```python
from build123d import *

# Parameters (mm, degrees)
BOSS_EXTRUDE1_DEPTH  = 46.3
SKETCH3_R            = 11.25
CUT_EXTRUDE2_DEPTH   = 2
SKETCH3_5_R          = 1.5
SKETCH3_5_R_2        = 3
CUT_EXTRUDE3_DEPTH   = 5
SKETCH4_R            = 2
CUT_EXTRUDE4_DEPTH   = 5
SKETCH5_W            = 5
SKETCH5_H            = 35.2
BOSS_EXTRUDE2_DEPTH  = 35.2
BOSS_EXTRUDE4_DEPTH  = 12
SKETCH8_R            = 2
SKETCH8_R_2          = 3
CUT_EXTRUDE5_DEPTH   = 5
SKETCH8_3_R          = 11
CUT_EXTRUDE6_DEPTH   = 2
SKETCH10_W           = 51.3
SKETCH10_H           = 12.4
BOSS_EXTRUDE8_DEPTH  = 5
SKETCH11_W           = 51.3
SKETCH11_H           = 12.4
BOSS_EXTRUDE9_DEPTH  = 5
BOSS_EXTRUDE10_DEPTH = 4
BOSS_EXTRUDE11_DEPTH = 4
SKETCH15_W           = 23.15
SKETCH15_H           = 6
CUT_EXTRUDE7_DEPTH   = 5
SKETCH18_R           = 3.5
BOSS_EXTRUDE12_DEPTH = 15


with BuildPart() as part:
    # Sketch1 → Boss-Extrude1 (new body)
    with BuildSketch(Plane(origin=(0, 0, 0), x_dir=(1, 0, 0), z_dir=(0, 1, 0))):
        Polygon((0, 0), (46.3, 0), (46.3, 50), (0, 50), (0, 55), (51.3, 55), (51.3, -5), (0, -5), align=None)
    extrude(amount=BOSS_EXTRUDE1_DEPTH)

    # Sketch3 → Cut-Extrude2 (cut)
    with BuildSketch(Plane.XY.offset(-50)):
        with Locations((23.15, 23.15)):
            Circle(SKETCH3_R)
    extrude(amount=-CUT_EXTRUDE2_DEPTH, mode=Mode.SUBTRACT)

    # Sketch3<5> → Cut-Extrude3 (cut)
    with BuildSketch(Plane.XY.offset(-50)):
        with Locations((38.65, 38.65)):
            Circle(SKETCH3_5_R)
        with Locations((7.65, 38.65)):
            Circle(SKETCH3_5_R)
        with Locations((7.65, 7.65)):
            Circle(SKETCH3_5_R)
        with Locations((38.65, 7.65)):
            Circle(SKETCH3_5_R)
        with Locations((23.15, 23.15)):
            Circle(SKETCH3_5_R_2)
    extrude(amount=-CUT_EXTRUDE3_DEPTH, mode=Mode.SUBTRACT)

    # Sketch4 → Cut-Extrude4 (cut)
    with BuildSketch(Plane(origin=(0, 0, 0), x_dir=(-1, 0, 0), z_dir=(0, 0, -1))):
        with Locations((-7.65, 7.65)):
            Circle(SKETCH4_R)
        with Locations((-7.65, 38.65)):
            Circle(SKETCH4_R)
        with Locations((-38.65, 7.65)):
            Circle(SKETCH4_R)
        with Locations((-38.65, 38.65)):
            Circle(SKETCH4_R)
    extrude(amount=-CUT_EXTRUDE4_DEPTH, mode=Mode.SUBTRACT)

    # Sketch5 → Boss-Extrude2 (add)
    with BuildSketch(Plane.XZ):
        with Locations((48.8, -25)):
            Rectangle(SKETCH5_W, SKETCH5_H)
    extrude(amount=BOSS_EXTRUDE2_DEPTH)

    # Sketch6 → Boss-Extrude4 (add)
    with BuildSketch(Plane(origin=(51.3, 0, 0), x_dir=(0, 0, -1), z_dir=(1, 0, 0))):
        Polygon((7.4, 0), (3.4, 0), (3.4, -39.2), (46.6, -39.2), (46.6, 0), (42.6, 0), (42.6, -35.2), (7.4, -35.2), align=None)
    extrude(amount=-BOSS_EXTRUDE4_DEPTH)

    # Sketch8 → Cut-Extrude5 (cut)
    with BuildSketch(Plane.ZY.offset(-46.3)):
        with Locations((-12, -4.6)):
            Circle(SKETCH8_R)
        with Locations((-38, -4.6)):
            Circle(SKETCH8_R)
        with Locations((-38, -30.6)):
            Circle(SKETCH8_R)
        with Locations((-12, -30.6)):
            Circle(SKETCH8_R)
        with Locations((-25, -17.6)):
            Circle(SKETCH8_R_2)
    extrude(amount=-CUT_EXTRUDE5_DEPTH, mode=Mode.SUBTRACT)

    # Sketch8<3> → Cut-Extrude6 (cut)
    with BuildSketch(Plane.ZY.offset(-46.3)):
        with Locations((-25, -17.6)):
            Circle(SKETCH8_3_R)
    extrude(amount=-CUT_EXTRUDE6_DEPTH, mode=Mode.SUBTRACT)

    # Sketch10 → Boss-Extrude8 (add)
    with BuildSketch(Plane.XZ):
        with Locations((25.65, -1.2)):
            Rectangle(SKETCH10_W, SKETCH10_H)
    extrude(amount=BOSS_EXTRUDE8_DEPTH)

    # Sketch11 → Boss-Extrude9 (add)
    with BuildSketch(Plane.XZ):
        with Locations((25.65, -48.8)):
            Rectangle(SKETCH11_W, SKETCH11_H)
    extrude(amount=BOSS_EXTRUDE9_DEPTH)

    # Sketch12 → Boss-Extrude10 (add)
    with BuildSketch(Plane.XY.offset(-42.6)):
        Polygon((39.3, -5), (14.3, -5), (39.3, -35.2), align=None)
    extrude(amount=-BOSS_EXTRUDE10_DEPTH)

    # Sketch13 → Boss-Extrude11 (add)
    with BuildSketch(Plane(origin=(0, 0, -7.4), x_dir=(-1, 0, 0), z_dir=(0, 0, -1))):
        Polygon((-39.3, -5), (-14.3, -5), (-39.3, -35.2), align=None)
    extrude(amount=-BOSS_EXTRUDE11_DEPTH)

    # Sketch15 → Cut-Extrude7 (cut)
    with BuildSketch(Plane(origin=(0, 0, -55), x_dir=(-1, 0, 0), z_dir=(0, 0, -1))):
        with Locations((-11.575, 23.15)):
            Rectangle(SKETCH15_W, SKETCH15_H)
    extrude(amount=-CUT_EXTRUDE7_DEPTH, mode=Mode.SUBTRACT)

    # Sketch18 → Boss-Extrude12 (add)
    with BuildSketch(Plane(origin=(0, 0, 0), x_dir=(-1, 0, 0), z_dir=(0, 0, -1))):
        with Locations((-23.15, 23.15)):
            Circle(SKETCH18_R)
    extrude(amount=-BOSS_EXTRUDE12_DEPTH)


solid = part.part
```
CAD build for the part. Positions are in the model's coordinates, mm. A direction names the side the tool comes from. Give positions to 0.01 mm unless a question says otherwise; leave off trailing zeros. Loops run counter-clockwise (first coordinate to the right, second up) from the corner with the lowest first, then second, coordinate; pieces in that order, holes last. Notation, with made-up numbers: (72.25, 25.5) -> (118.25, 25.5) arc R25 cw to (118.25, 42.5) -> close; hole circle Ø9 at (6.5, -16.5). An arc over 180 degrees is marked (long way). Use a Markdown table: item, result.
1. Slice it at A-A (y = 38.65). List the corners of the cut face in (x, z).
Check result:
| item | result |
|---|---|
| outline | (0, -55) -> (6.15, -55) -> (6.15, -50) -> (0, -50) -> close; (0, 0) -> (5.65, 0) -> (5.65, 5) -> (0, 5) -> close; (9.15, -55) -> (37.15, -55) -> (37.15, -50) -> (9.15, -50) -> close; (9.65, 0) -> (36.65, 0) -> (36.65, 5) -> (9.65, 5) -> close; (40.15, -55) -> (51.3, -55) -> (51.3, 5) -> (40.65, 5) -> (40.65, 0) -> (46.3, 0) -> (46.3, -50) -> (40.15, -50) -> close |
2. Which spindle directions (+Z, -Z, +X, -X, +Y, -Y) get a long thin tool onto all of the face, cutting with end or side? Do faces 4 (the cylindrical face through (26.15, 23.08, -53.48)), 5 (the flat face through (39.3, -37, -25)), 6 (the flat face through (23, 23, 0)). Say none if no direction does.
Check result:
| item | result |
|---|---|
| face 4 | -Z, -X |
| face 5 | +Z, -Z, -X, -Y |
| face 6 | -X, +Y |
3. Wall check: L1, parallel to Y at x = 7.65, z = 2.2; L2, parallel to X at y = 38, z = 1; L3, parallel to Z at x = 21.5, y = 17.5. Give the ranges that are in metal, low to high. Write a range as [from, to].
Check result:
| item | result |
|---|---|
| L1 | y = [-5, 5.65], [9.65, 36.65], [40.65, 46.3] |
| L2 | x = [0, 5.76], [9.54, 36.76], [40.54, 51.3] |
| L3 | z = [-55, -52], [0, 5] |
4. Slice it at B-B (x = 7.65). Give the number of separate pieces and of enclosed holes in the cut face, plus the area to 3 significant figures.
Check result:
| item | result |
|---|---|
| separate pieces | 7 |
| enclosed holes | 0 |
| area | 487 mm^2 |
5. Flat gauge pins, fed straight in: pin 1 (4.5 mm diameter, centred on y = -37.5, z = -33.5, fed in from -X); pin 2 (6.5 mm diameter, centred on y = -4.6, z = -38, fed in from -X); pin 3 (3.5 mm diameter, centred on x = 38.65, y = 7.65, fed in from +Z). Where does each tip first touch, or does it go through?
Check result:
| item | result |
|---|---|
| pin 1 | stops at x = 39.3 |
| pin 2 | stops at x = 46.3 |
| pin 3 | stops at z = -50 |
6. Mould opens along X. For faces 1 (the cylindrical face through (34.39, 22.7, -50.99)), 2 (the flat face through (34, 18, -50)), 3 (the cylindrical face through (25.73, 25.515, 9.93)) say: pulls with the +X half, pulls with the -X half, needs draft (parallel to the pull), parting line crosses it, or undercut.
Check result:
| item | result |
|---|---|
| face 1 | undercut |
| face 2 | needs draft |
| face 3 | parting line crosses it |
7. Slice it at D-D (y = 23.15). List the corners of the cut face in (x, z).
Check result:
| item | result |
|---|---|
| outline | (0, 0) -> (46.3, 0) -> (46.3, -50) -> (34.4, -50) -> (34.4, -52) -> (26.15, -52) -> (26.15, -55) -> (51.3, -55) -> (51.3, 5) -> (26.65, 5) -> (26.65, 15) -> (19.65, 15) -> (19.65, 5) -> (0, 5) -> close |
8. Slice it at C-C (z = -12). List the corners of the cut face in (x, y), plus the area to 4 significant figures.
Check result:
| item | result |
|---|---|
| outline | (39.3, -39.2) -> (51.3, -39.2) -> (51.3, -32.6) -> (46.3, -32.6) -> (46.3, -35.2) -> (39.3, -35.2) -> close; (46.3, -28.6) -> (51.3, -28.6) -> (51.3, -6.6) -> (46.3, -6.6) -> close; (46.3, -2.6) -> (51.3, -2.6) -> (51.3, 46.3) -> (46.3, 46.3) -> close |
| area | 415.5 mm^2 |
